Check sheet for the modelled part. Datum: model origin and axes. Units: mm. Face numbers are marked on the shaded views. Coordinates: 2 decimals unless noted, no trailing zeros. Loops run counter-clockwise (first coordinate to the right, second up) from the corner with the lowest first, then second, coordinate; pieces in that order, holes last. Notation, with made-up numbers: M 39,-4 L 96,-4 A34 cw 96,29 Z; hole C 86.5,11.25 d2. An arc over 180 degrees is marked long. Write each question's results on one line, items separated by ' | '. Start each with the question number.
from build123d import *

# Parameters (mm, degrees)
SKETCH1_R           = 2.5
BOSS_EXTRUDE1_DEPTH = 10
SKETCH2_R           = 30.5
SKETCH2_R_2         = 19.5
CUT_EXTRUDE1_DEPTH  = 4
SKETCH3_R           = 17.5
BOSS_EXTRUDE2_DEPTH = 4


with BuildPart() as part:
    # Sketch1 → Boss-Extrude1 (new body)
    with BuildSketch(Plane(origin=(0, 0, 0), x_dir=(1, 0, 0), z_dir=(0, 1, 0))):
        with BuildLine():
            Line((-99.5, 86.5), (99.5, 86.5))
            ThreePointArc((99.5, 86.5), (107.985281374, 82.985281374), (111.5, 74.5))
            Line((111.5, 74.5), (111.5, -74.5))
            ThreePointArc((111.5, -74.5), (107.985281374, -82.985281374), (99.5, -86.5))
            Line((99.5, -86.5), (-99.5, -86.5))
            ThreePointArc((-99.5, -86.5), (-107.985281374, -82.985281374), (-111.5, -74.5))
            Line((-111.5, -74.5), (-111.5, 74.5))
            ThreePointArc((-111.5, 74.5), (-107.985281374, 82.985281374), (-99.5, 86.5))
        make_face()
        with Locations(Location((100, 75, 0), (0, 0, 270))):
            Circle(SKETCH1_R, mode=Mode.SUBTRACT)
        with Locations(Location((100, -75, 0), (0, 0, 270))):
            Circle(SKETCH1_R, mode=Mode.SUBTRACT)
        with Locations(Location((-100, -75, 0), (0, 0, 270))):
            Circle(SKETCH1_R, mode=Mode.SUBTRACT)
        with Locations(Location((-100, 75, 0), (0, 0, 270))):
            Circle(SKETCH1_R, mode=Mode.SUBTRACT)
    extrude(amount=-BOSS_EXTRUDE1_DEPTH)

    # Sketch2 → Cut-Extrude1 (cut)
    with BuildSketch(Plane(origin=(0, 0, 0), x_dir=(1, 0, 0), z_dir=(0, 1, 0))):
        with Locations(Location((0, 0, 0), (0, 0, 270))):
            Circle(SKETCH2_R)
        with Locations(Location((0, 0, 0), (0, 0, 270))):
            Circle(SKETCH2_R_2, mode=Mode.SUBTRACT)
    extrude(amount=-CUT_EXTRUDE1_DEPTH, mode=Mode.SUBTRACT)

    # Sketch3 → Boss-Extrude2 (add)
    with BuildSketch(Plane(origin=(0, 0, 0), x_dir=(1, 0, 0), z_dir=(0, 1, 0))):
        with Locations(Location((0, 0, 0), (0, 0, 270))):
            Circle(SKETCH3_R)
    extrude(amount=BOSS_EXTRUDE2_DEPTH)


solid = part.part
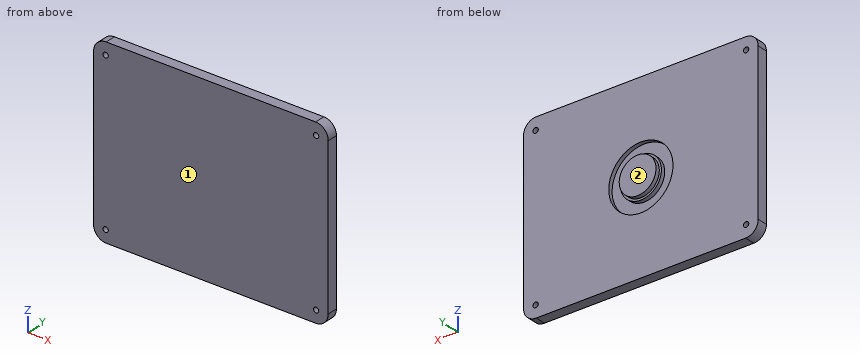
1) Section check D-D (z = 43). Enter the section's corners in (x, y).
2) Section check A-A (x = 0). Enter the section's corners in (y, z).
3) Gauge pin test, flat end, axial feed: P1, Ø6.5, axis at x = 100, z = -75, coming from the +Y side. Record the tip position at first contact, or that the pin passes through.
4) Release check for a two-part mould opening along Y. For the marked faces 1 and 2 record: +Y half, -Y half, draft (parallel to the pull), parting line (faces both ways), or undercut.
5) Section check C-C (x = 50). Enter the section's corners in (y, z), then the cut area to 3 significant figures.
6) Thickness scan on probe 1 along X at (y, z) = (-1.35, 0); probe 2 along X at (y, z) = (-6.75, 75); probe 3 along Y at (x, z) = (23, 33.5). Record the ranges inside material, lowest first.
7) Section check B-B (z = 0). Enter the section's corners in (x, y).
Return value:
1) outline: M -111.5,-10 L 111.5,-10 L 111.5,0 L -111.5,0 Z
2) outline: M -10,-86.5 L 0,-86.5 L 0,-30.5 L -4,-30.5 L -4,-19.5 L 0,-19.5 L 0,-17.5 L 4,-17.5 L 4,17.5 L 0,17.5 L 0,19.5 L -4,19.5 L -4,30.5 L 0,30.5 L 0,86.5 L -10,86.5 Z
3) P1: stops at y = 0
4) face 1: -Y half | face 2: +Y half
5) outline: M -10,-86.5 L 0,-86.5 L 0,86.5 L -10,86.5 Z | area: 1,730 mm2
6) probe 1: x = -111.5 to -30.5, -19.5 to 19.5, 30.5 to 111.5 | probe 2: x = -111.49 to -102.5, -97.5 to 97.5, 102.5 to 111.49 | probe 3: y = -10 to 0
7) outline: M -111.5,-10 L 111.5,-10 L 111.5,0 L 30.5,0 L 30.5,-4 L 19.5,-4 L 19.5,0 L 17.5,0 L 17.5,4 L -17.5,4 L -17.5,0 L -19.5,0 L -19.5,-4 L -30.5,-4 L -30.5,0 L -111.5,0 Z
